Verification items for the finished model (mm, model axes). A direction names the side the tool comes from. Round coordinates to 2 decimals unless told otherwise and drop trailing zeros. Write each loop counter-clockwise with the first axis right and the second up, starting at its lowest first coordinate (ties: lowest second). Pieces come first, ordered by that corner, then holes. Notation, with made-up numbers: M 80,-2 L 105,-2 A27 cw 105,23 Z; hole C 7,11 d11. An arc over 180 degrees is marked long. Answer in a Markdown table with one row per item. Add a question column.
1. Sectioned sample at A-A on x = 3. Record the cut outline in (y, z).
2. Sectioned sample at B-B on x = -13.65. Record the cut outline in (y, z).
3. Sectioned sample at D-D on z = -4.75. Record the cut outline in (x, y).
4. Draft check along Z on faces 5 (the flat face through (2, 13, -2.5)), 6 (the flat face through (15, 6, -0.65)), 7 (the cylindrical face through (5.95, 13.32, 0.05)), 8 (the flat face through (11.25, -4, 0)). Enter one of: pulls with the +Z half, pulls with the -Z half, needs draft (parallel to the pull), parting line crosses it, or undercut.
5. Go/stop test with flat-tipped pins: pin 1 Ø3 at (x, z) = (-13.65, 0) entering from -Y; pin 2 Ø1.5 at (x, z) = (-5.35, 0) entering from +Y; pin 3 Ø1.9 at (x, z) = (-5, 0) entering from +Y; pin 4 Ø3 at (x, y) = (1, 13) entering from -Z. Record where each tip stops, or that it passes through.
6. Sectioned sample at C-C on y = 6.25. Record the cut outline in (x, z), plus the area to 3 significant figures.
7. Material ranges on probe 1 along Z at (x, y) = (-13.65, 5.65); probe 2 along X at (y, z) = (17.6, 0); probe 3 along Z at (x, y) = (-5.35, 16.35), recorded low to high.
8. Set-up check for faces 1 (the flat face through (-11.25, 9, 0)), 2 (the cylindrical face through (-6.02, 16.93, 0.52)), 3 (the flat face through (-15, 6, 0.65)), 4 (the flat face through (12.5, 4.55, -0.1)): record each of +Z, -Z, +X, -X, +Y, -Y from which the full face is reachable in a straight line by a thin tool's end or side.
```python
from build123d import *

# Parameters (mm, degrees)
SKETCH2_W           = 22.5
SKETCH2_H           = 22.7
BOSS_EXTRUDE1_DEPTH = 5.9
BOSS_EXTRUDE2_DEPTH = 2.5
BOSS_EXTRUDE3_DEPTH = 4
SKETCH5_R           = 2.3
SKETCH5_R_2         = 0.85
BOSS_EXTRUDE4_DEPTH = 3.2


with BuildPart() as part:
    # Sketch2 → Boss-Extrude1 (new body, symmetric)
    with BuildSketch(Plane.XY):
        Rectangle(SKETCH2_W, SKETCH2_H)
    extrude(amount=BOSS_EXTRUDE1_DEPTH, both=True)

    # Sketch3 → Boss-Extrude2 (add)
    with BuildSketch(Plane(origin=(0, 4.55, 0), x_dir=(-1, 0, 0), z_dir=(0, -1, 0))):
        with BuildLine():
            Line((14.409934208, 0.65), (15.95, 0.65))
            Line((15.95, 0.65), (15.95, 5.9))
            Line((15.95, 5.9), (11.25, 5.9))
            Line((11.25, 5.9), (11.25, -5.9))
            Line((11.25, -5.9), (15.95, -5.9))
            Line((15.95, -5.9), (15.95, -0.65))
            Line((15.95, -0.65), (14.409934208, -0.65))
            ThreePointArc((14.409934208, -0.65), (12.65, 0), (14.409934208, 0.65))
        make_face()
        with BuildLine():
            Line((-11.25, -5.9), (-15.95, -5.9))
            Line((-15.95, -5.9), (-15.95, -0.65))
            Line((-15.95, -0.65), (-14.409934208, -0.65))
            ThreePointArc((-14.409934208, -0.65), (-12.65, 0), (-14.409934208, 0.65))
            Line((-14.409934208, 0.65), (-15.95, 0.65))
            Line((-15.95, 0.65), (-15.95, 5.9))
            Line((-15.95, 5.9), (-11.25, 5.9))
            Line((-11.25, 5.9), (-11.25, -5.9))
        make_face()
    extrude(amount=-BOSS_EXTRUDE2_DEPTH)

    # Sketch4 → Boss-Extrude3 (add)
    with BuildSketch(Plane(origin=(0, 11.35, 0), x_dir=(1, 0, 0), z_dir=(0, 1, 0))):
        with BuildLine():
            Line((3.45, 2.5), (-0.005844314, 2.5))
            ThreePointArc((-0.005844314, 2.5), (-11.25, 0), (-0.005844314, -2.5))
            Line((-0.005844314, -2.5), (3.45, -2.5))
            ThreePointArc((3.45, -2.5), (5.95, 0), (3.45, 2.5))
        make_face()
    extrude(amount=BOSS_EXTRUDE3_DEPTH)

    # Sketch5 → Boss-Extrude4 (add)
    with BuildSketch(Plane(origin=(0, 15.35, 0), x_dir=(1, 0, 0), z_dir=(0, 1, 0))):
        with Locations((-5.35, 0)):
            Circle(SKETCH5_R)
        with Locations((-5.35, 0)):
            Circle(SKETCH5_R_2, mode=Mode.SUBTRACT)
    extrude(amount=BOSS_EXTRUDE4_DEPTH)


solid = part.part
```
Geometry check:
| question | item | result |
|---|---|---|
| 1 | outline | M -11.35,-5.9 L 11.35,-5.9 L 11.35,-2.5 L 15.35,-2.5 L 15.35,2.5 L 11.35,2.5 L 11.35,5.9 L -11.35,5.9 Z |
| 2 | outline | M 4.55,-5.9 L 7.05,-5.9 L 7.05,-1 L 4.55,-1 Z; M 4.55,1 L 7.05,1 L 7.05,5.9 L 4.55,5.9 Z |
| 3 | outline | M -15.95,4.55 L -11.25,4.55 L -11.25,-11.35 L 11.25,-11.35 L 11.25,4.55 L 15.95,4.55 L 15.95,7.05 L 11.25,7.05 L 11.25,11.35 L -1.85,11.35 L -1.85,15.35 L -8.85,15.35 L -8.85,11.35 L -11.25,11.35 L -11.25,7.05 L -15.95,7.05 Z |
| 4 | face 5 | pulls with the -Z half |
| 4 | face 6 | undercut |
| 4 | face 7 | parting line crosses it |
| 4 | face 8 | needs draft |
| 5 | pin 1 | stops at y = 4.55 |
| 5 | pin 2 | stops at y = 15.35 |
| 5 | pin 3 | stops at y = 18.55 |
| 5 | pin 4 | stops at z = -3.36 |
| 6 | outline | M -15.95,-5.9 L 15.95,-5.9 L 15.95,-0.65 L 14.41,-0.65 A1 cw long 14.41,0.65 L 15.95,0.65 L 15.95,5.9 L -15.95,5.9 L -15.95,0.65 L -14.41,0.65 A1 cw long -14.41,-0.65 L -15.95,-0.65 Z |
| 6 | area | 367 mm2 |
| 7 | probe 1 | z = -5.9 to -1, 1 to 5.9 |
| 7 | probe 2 | x = -7.65 to -6.2, -4.5 to -3.05 |
| 7 | probe 3 | z = -2.3 to -0.85, 0.85 to 2.3 |
| 8 | face 1 | +Z, -Z, -X, +Y |
| 8 | face 2 | +Y |
| 8 | face 3 | -X, +Y, -Y |
| 8 | face 4 | +Z, -Z, +X, -Y |
